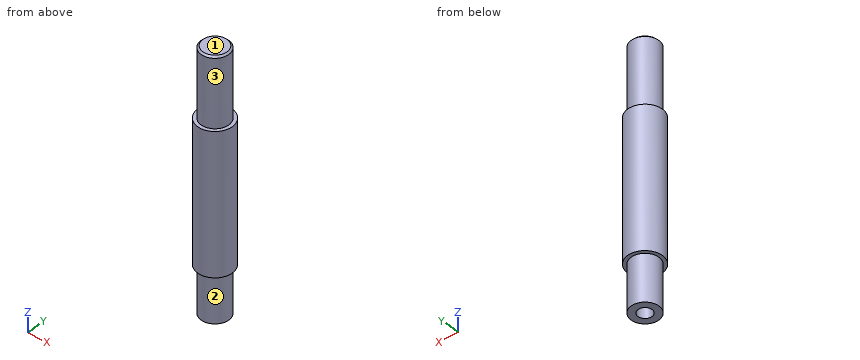
```python
from build123d import *

# Parameters (mm, degrees)
CROQUIS1_R              = 8
SALIENTE_EXTRUIR1_DEPTH = 27
CROQUIS2_R              = 10
SALIENTE_EXTRUIR2_DEPTH = 81
CROQUIS3_R              = 8
SALIENTE_EXTRUIR3_DEPTH = 40
CHAFL_N1_SIZE           = 1
CROQUIS4_R              = 4
CORTAR_EXTRUIR1_DEPTH   = 25


with BuildPart() as part:
    # Croquis1 → Saliente-Extruir1 (new body)
    with BuildSketch(Plane.XY):
        Circle(CROQUIS1_R)
    extrude(amount=SALIENTE_EXTRUIR1_DEPTH)

    # Croquis2 → Saliente-Extruir2 (add)
    with BuildSketch(Plane.XY.offset(27)):
        Circle(CROQUIS2_R)
    extrude(amount=SALIENTE_EXTRUIR2_DEPTH)

    # Croquis3 → Saliente-Extruir3 (add)
    with BuildSketch(Plane.XY.offset(108)):
        Circle(CROQUIS3_R)
    extrude(amount=SALIENTE_EXTRUIR3_DEPTH)

    # Chaflán1
    chafl_n1_edges = [part.edges().sort_by_distance(p)[0] for p in [
        (-8, 0, 148),
    ]]
    chamfer(chafl_n1_edges, length=CHAFL_N1_SIZE)

    # Croquis4 → Cortar-Extruir1 (cut)
    with BuildSketch(Plane(origin=(0, 0, 0), x_dir=(-1, 0, 0), z_dir=(0, 0, -1))):
        Circle(CROQUIS4_R)
    extrude(amount=-CORTAR_EXTRUIR1_DEPTH, mode=Mode.SUBTRACT)


solid = part.part
```
CAD build for the part. Positions are in the model's coordinates, mm. Face numbers are marked on the shaded views. A direction names the side the tool comes from. Coordinates: 2 decimals unless noted, no trailing zeros. Write each loop counter-clockwise with the first axis right and the second up, starting at its lowest first coordinate (ties: lowest second). Pieces come first, ordered by that corner, then holes. Notation, with made-up numbers: (53.5, 3) -> (79.5, 3) arc R24 cw to (79.5, 19) -> close; hole circle Ø2 at (12.5, -6). An arc over 180 degrees is marked (long way). Use CSV: the item, a comma, the result in double quotes. Start each with the question number.
Item 1: Band-saw the part on A-A, the plane y = 0. Write the cut outline in (x, z).
Item 2: Wall check: probe 1 along Y at (x, z) = (0, 12.5); probe 2 along Y at (x, z) = (0, 129); probe 3 along Z at (x, y) = (6, -7). Give the ranges that are in metal, low to high.
Item 3: Tool access for the marked faces 1, 2 and 3: list every direction of +Z, -Z, +X, -X, +Y, -Y with a clear straight run to the whole face (end or side of a thin tool).
Item 4: Drop flat-ended pins along their axis: P1, Ø1.5, axis at x = 0, y = 3.5, coming from the -Z side; P2, Ø2.5, axis at x = -2, y = 1.5, coming from the -Z side; P3, Ø2, axis at x = -4.5, z = 86, coming from the +Y side; P4, Ø8, axis at y = 3, z = 127, coming from the -X side. Give the stop position or say it passes through.
Item 5: Band-saw the part on C-C, the plane z = 95. Write the cut outline in (x, y), plus the area to 3 significant figures.
Response values:
1,outline,"(-10, 27) -> (-8, 27) -> (-8, 0) -> (-4, 0) -> (-4, 25) -> (4, 25) -> (4, 0) -> (8, 0) -> (8, 27) -> (10, 27) -> (10, 108) -> (8, 108) -> (8, 147) -> (7, 148) -> (-7, 148) -> (-8, 147) -> (-8, 108) -> (-10, 108) -> close"
2,probe 1,"y = -8 to -4, 4 to 8"
2,probe 2,"y = -8 to 8"
2,probe 3,"z = 27 to 108"
3,face 1,"+Z, +X, -X, +Y, -Y"
3,face 2,"-Z"
3,face 3,"+Z"
4,P1,"stops at z = 0"
4,P2,"stops at z = 25"
4,P3,"stops at y = 9.37"
4,P4,"stops at x = -8"
5,outline,"circle Ø20 at (0, 0)"
5,area,"314 mm2"
